Autodesk Inventor part; units mm, degrees
ref_plane "YZ Plane" through (0, 0, 0) normal (1, 0, 0) x (0, 1, 0)
ref_plane "XZ Plane" through (0, 0, 0) normal (0, 1, 0) x (-1, 0, 0)
ref_plane "XY Plane" through (0, 0, 0) normal (0, 0, 1) x (1, 0, 0)
sketch "Sketch1" plane through (0, 0, 0) normal (1, 0, 0) x (0, 1, 0)
  line L0 (0, 0) -> (57.15, 0)
  line L1 (57.15, 0) -> (57.15, 193.675)
  line L2 (57.15, 193.675) -> (0, 193.675)
  line L3 (0, 193.675) -> (0, 0)
  dimension "d0" = 57.15
  dimension "d1" = 193.675
extrude "Extrusion1" add sketch "Sketch1" along normal blind 477.8375
sketch "Sketch3" plane through (0, 0, 0) normal (0, 0, -1) x (-1, 0, 0)
  line L0 (-477.8375, 0) -> (-397.0152, 0) construction
  line L1 (-477.8375, 57.15) -> (-477.8375, 0)
  line L2 (0, 0) -> (-477.8375, 0)
  line L3 (-477.8375, 57.15) -> (-420.6875, 0)
  line L4 (-477.8375, 57.15) -> (-477.8375, 0)
  line L5 (-477.8375, 0) -> (-420.6875, 0)
extrude "Extrusion3" cut sketch "Sketch3" against normal up to surface (193.675 mm away)
thicken "Thicken1" operation add thickness 3.175 both sides no extend neighbours yes toward (-0.7071068, 0.7071068, 0) faces at (458.7875, 38.1, 129.1167)
sketch "Sketch4" plane through (0, 0, 0) normal (0, 0, -1) x (-1, 0, 0)
  line L0 (0, 57.15) -> (-473.3474, 57.15)
  line L1 (-460.6474, 57.15) -> (-460.6474, 44.45)
  line L2 (-473.3474, 57.15) -> (-416.1974, 0)
  line L3 (-473.3474, 57.15) -> (-460.6474, 57.15)
  line L4 (-460.6474, 44.45) -> (-473.3474, 57.15)
  point P0 (0, 0)
  dimension "d17" = 12.7
extrude "Extrusion4" cut sketch "Sketch4" against normal blind 193.675
sketch "Sketch6" plane through (0, 0, 0) normal (-1, 0, 0) x (0, 0, 1)
  line L0 (0, 57.15) -> (193.675, 57.15)
  line L1 (0, 0) -> (193.675, 0)
  line L2 (193.675, 0) -> (193.675, 57.15)
  line L3 (193.675, 57.15) -> (0, 57.15)
  line L4 (0, 57.15) -> (0, 0)
extrude "Extrusion5" add sketch "Sketch6" along normal blind 17.1831
properties part number "1-80" material "Granite, Cut, Polished"
CAD build for the part. Positions are in the model's coordinates, mm. Coordinates: 2 decimals unless noted, no trailing zeros. Write each loop counter-clockwise with the first axis right and the second up, starting at its lowest first coordinate (ties: lowest second). Pieces come first, ordered by that corner, then holes. Notation, with made-up numbers: (77, -8) -> (118, -8) arc R23 cw to (118, 0) -> close; hole circle Ø1 at (38, 9.5). An arc over 180 degrees is marked (long way). Use CSV: the item, a comma, the result in double quotes. Start each with the question number.
Item 1: Drop a flat-ended pin along its axis: P1, Ø12, axis at x = 325, z = 84.5, coming from the -Y side. Give the stop position or say it passes through.
Item 2: Wall check: probe 1 along X at (y, z) = (5, 118); probe 2 along X at (y, z) = (42.5, 57.5). Give the ranges that are in metal, low to high.
Item 3: Band-saw the part on B-B, the plane y = 6.5. Write the cut outline in (x, z) (3 decimals).
Item 4: Band-saw the part on C-C, the plane y = 26.5. Write the cut outline in (x, z) (3 decimals), plus the area to 3 significant figures.
Item 5: Band-saw the part on A-A, the plane z = 75. Write the cut outline in (x, y), plus the area to 3 significant figures.
Response values:
1,P1,"stops at y = 0"
2,probe 1,"x = -17.18 to 421.2"
2,probe 2,"x = -17.18 to 458.7"
3,outline,"(-17.183, 0) -> (422.697, 0) -> (422.697, 193.675) -> (-17.183, 193.675) -> close"
4,outline,"(-17.183, 0) -> (442.697, 0) -> (442.697, 193.675) -> (-17.183, 193.675) -> close"
4,area,"89,100 mm2"
5,outline,"(-17.18, 0) -> (416.2, 0) -> (460.65, 44.45) -> (460.65, 57.15) -> (-17.18, 57.15) -> close"
5,area,"26,300 mm2"
